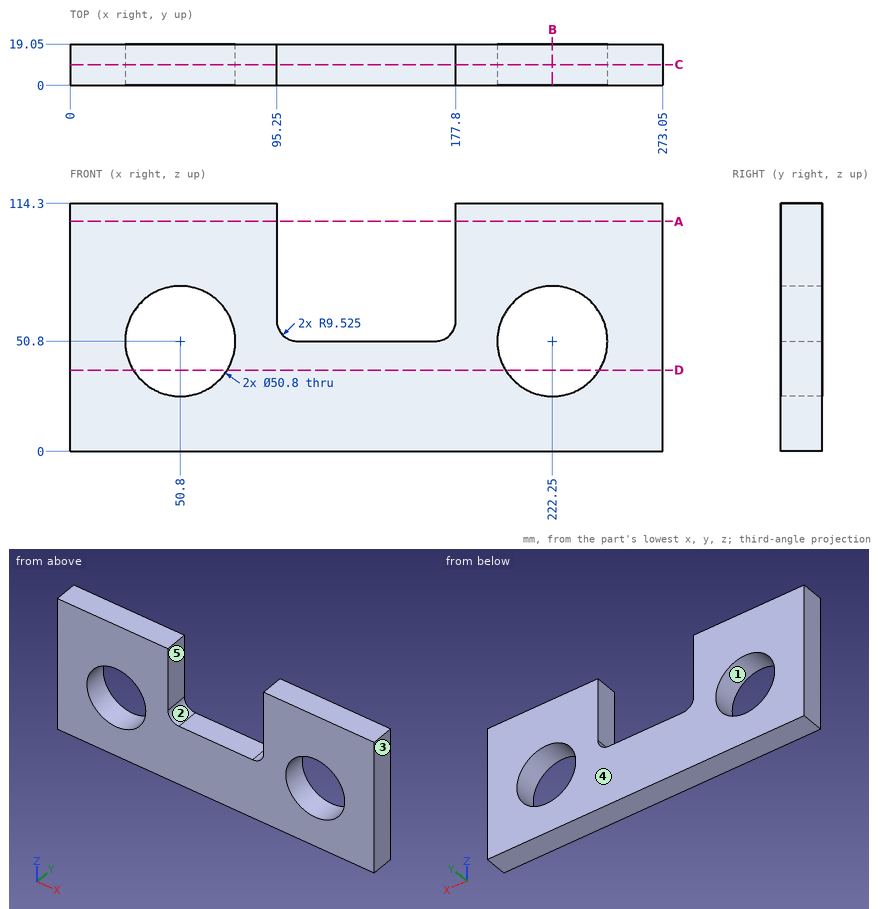
Job drawing, mm, ordinate dimensions from the low corner. One solid piece. A direction names the side the tool comes from. Round coordinates to 2 decimals unless told otherwise and drop trailing zeros. Loops run counter-clockwise (first coordinate to the right, second up) from the corner with the lowest first, then second, coordinate; pieces in that order, holes last. Notation, with made-up numbers: (80, 85) -> (99, 85) arc R16 ccw to (99, 94) -> close; hole circle Ø3 at (-3.5, -15.75). An arc over 180 degrees is marked (long way). One line per item, written item: value. Start each with the question number.
Q1. Probe line 1 along Z through (x, y) = (222.25, 8.25); line 2 along X through (y, z) = (7.75, 33.5); line 3 along X through (y, z) = (4.25, 63). List the from-to ranges inside material, lowest first.
Q2. Cut at B-B on x = 222.25. List the corners of the cut face in (y, z), plus the area to 3 significant figures.
Q3. Cut at A-A on z = 106. List the corners of the cut face in (x, y).
Q4. Cut at C-C on y = 9.5. List the corners of the cut face in (x, z) (3 decimals), plus the area to 3 significant figures.
Q5. Cut at D-D on z = 37.5. List the corners of the cut face in (x, y).
Q6. 3-axis set-ups, long thin cutter, end or side, ignore diameter. For the marked faces 4 and 5: which of +Z, -Z, +X, -X, +Y, -Y reach the whole face in a straight line?
Q7. Drop flat-ended pins along their axis: pin 1 Ø8 at (x, z) = (81, 46) entering from -Y; pin 2 Ø9.5 at (x, y) = (149.5, 11.5) entering from +Z. Give the stop position or say it passes through.
Q8. Two-plate mould, pull along Z, no slides. Class the marked faces 1, 2 and 3: released by +Z, released by -Z, zero draft, split by the parting line, or undercut.
Computed:
1. line 1: 0 to 25.4, 76.2 to 114.3
1. line 2: 0 to 32.2, 69.4 to 203.65, 240.85 to 273.05
1. line 3: 0 to 28.52, 73.08 to 95.25, 177.8 to 199.97, 244.53 to 273.05
2. outline: (0, 0) -> (19.05, 0) -> (19.05, 25.4) -> (0, 25.4) -> close; (0, 76.2) -> (19.05, 76.2) -> (19.05, 114.3) -> (0, 114.3) -> close
2. area: 1,210 mm²
3. outline: (0, 0) -> (95.25, 0) -> (95.25, 19.05) -> (0, 19.05) -> close; (177.8, 0) -> (273.05, 0) -> (273.05, 19.05) -> (177.8, 19.05) -> close
4. outline: (0, 0) -> (273.05, 0) -> (273.05, 114.3) -> (177.8, 114.3) -> (177.8, 60.325) arc R9.525 cw to (168.275, 50.8) -> (104.775, 50.8) arc R9.525 cw to (95.25, 60.325) -> (95.25, 114.3) -> (0, 114.3) -> close; hole circle Ø50.8 at (50.8, 50.8); hole circle Ø50.8 at (222.25, 50.8)
4. area: 22,000 mm²
5. outline: (0, 0) -> (29.16, 0) -> (29.16, 19.05) -> (0, 19.05) -> close; (72.44, 0) -> (200.61, 0) -> (200.61, 19.05) -> (72.44, 19.05) -> close; (243.89, 0) -> (273.05, 0) -> (273.05, 19.05) -> (243.89, 19.05) -> close
6. face 4: +Z, -Z, +X, -X, +Y
6. face 5: +Z, +Y, -Y
7. pin 1: y = 0
7. pin 2: z = 50.8
8. face 1: undercut
8. face 2: released by +Z
8. face 3: zero draft
